Source: CAD feature listing. Evaluate the final solid. Frame: model axes, mm. Give positions to 0.01 mm unless a question says otherwise; leave off trailing zeros. Loops run counter-clockwise (first coordinate to the right, second up) from the corner with the lowest first, then second, coordinate; pieces in that order, holes last.
from build123d import *

# Parameters (mm, degrees)
SKETCH1_R           = 69.85
BOSS_EXTRUDE1_DEPTH = 6.35
SKETCH5_R           = 2.238375
SKETCH5_R_2         = 3.825875
CUT_EXTRUDE3_DEPTH  = 12.7


with BuildPart() as part:
    # Sketch1 → Boss-Extrude1 (new body)
    with BuildSketch(Plane(origin=(0, 0, 0), x_dir=(1, 0, 0), z_dir=(0, 1, 0))):
        with Locations(Location((-16.072515175, 12.054386381, 0), (0, 0, 270))):
            Circle(SKETCH1_R)
    extrude(amount=BOSS_EXTRUDE1_DEPTH)

    # Sketch5 → Cut-Extrude3 (cut)
    with BuildSketch(Plane(origin=(0, 6.35, 0), x_dir=(1, 0, 0), z_dir=(0, 1, 0))):
        with Locations(Location((-0.738778166, 69.280671968, 0), (0, 0, 270))):
            Circle(SKETCH5_R)
        with Locations(Location((-16.072515175, 56.504386381, 0), (0, 0, 270))):
            Circle(SKETCH5_R)
        with Locations(Location((-16.072515175, 12.054386381, 0), (0, 0, 270))):
            Circle(SKETCH5_R_2)
        with Locations(Location((-16.072515175, -32.395613619, 0), (0, 0, 270))):
            Circle(SKETCH5_R)
        with Locations(Location((-0.679642183, -45.392597698, 0), (0, 0, 270))):
            Circle(SKETCH5_R)
        with Locations(Location((41.966484825, 12.054386381, 0), (0, 0, 270))):
            Circle(SKETCH5_R)
    extrude(amount=-CUT_EXTRUDE3_DEPTH, mode=Mode.SUBTRACT)


solid = part.part
1) Pull-direction query (X, two-part tool) for faces 1 (the flat face through (-31, 6.35, -13)), 2 (the cylindrical face through (-0.581, 3.219, 43.156)), 3 (the cylindrical face through (-58.58, 3.13, -67.48)); classes: released by +X, released by -X, zero draft, split by the parting line, or undercut.
Checks:
face 1: zero draft
face 2: undercut
face 3: split by the parting line
2) Cut plane D-D (z = 1). Return loops of the section in (x, y).
Checks:
outline: (-84.69, 0) - (52.55, 0) - (52.55, 6.35) - (-84.69, 6.35) - close
3) Cut plane C-C (x = -60). Return loops of the section in (y, z).
Checks:
outline: (0, -66.36) - (6.35, -66.36) - (6.35, 42.25) - (0, 42.25) - close
4) Cut plane B-B (y = 2.25). Return loops of the section in (x, z).
Checks:
outline: circle Ø139.7 at (-16.07, -12.05); hole circle Ø7.65 at (-16.07, -12.05); hole circle Ø4.48 at (-16.07, -56.5); hole circle Ø4.48 at (-16.07, 32.4); hole circle Ø4.48 at (-0.74, -69.28); hole circle Ø4.48 at (-0.68, 45.39); hole circle Ø4.48 at (41.97, -12.05)
5) Cut plane A-A (z = -69.5). Return loops of the section in (x, y).
Checks:
outline: (-55.81, 0) - (-2.97, 0) - (-2.97, 6.35) - (-55.81, 6.35) - close; (1.49, 0) - (23.66, 0) - (23.66, 6.35) - (1.49, 6.35) - close
6) Contact query for flat-ended pins moving along their axis: P1, Ø2.5, axis at x = -0.74, z = -69.28, coming from the +Y side; P2, Ø1, axis at x = -24, y = 1, coming from the +Z side. Output: stop coordinate, or through.
Checks:
P1: passes through
P2: stops at z = 57.4
7) Ray query, probe 1 along X at (y, z) = (5.25, -13.5); probe 2 along X at (y, z) = (2.75, 33.5); probe 3 along Z at (x, y) = (21.5, 2.5). Return the intervals inside material, ascending.
Checks:
probe 1: x = -85.91 to -19.61, -12.53 to 40.26, 43.68 to 53.76
probe 2: x = -69.02 to -18.02, -14.13 to 36.88
probe 3: z = -70.94 to 46.83
